Design review of the part built by this model. Coordinates are the model's own, in mm. A direction names the side the tool comes from. Coordinates: 2 decimals unless noted, no trailing zeros. Order: outer loops, then holes, each group sorted by start corner. A loop starts at its lowest first (then second) coordinate and runs counter-clockwise, first axis right, second up. Notation, with made-up numbers: (86, 62.25) -> (104, 62.25) arc R23 ccw to (104, 96.25) -> close; hole circle Ø7 at (6.25, -15). An arc over 180 degrees is marked (long way). Use a Markdown table: item, result. Add a question column.
Q1. Machinability: for faces 4 (the face through (-98.827, 0, 8)), 5 (the face through (-91.827, 0, 12)), which of the approach directions +Z, -Z, +X, -X, +Y, -Y give a long, thin tool a straight path to every point of the face, cutting with its end or side? Answer none if there is none.
Q2. Add section C-C (x = -59.5). State the section outline as (y, z) points, then the cut area to 4 significant figures.
Q3. Add section A-A (z = 12.25). State the section outline as (x, y) points, then the cut area to 4 significant figures.
Q4. Wall thickness on probe 1 along X at (y, z) = (1.5, 8); probe 2 along Z at (x, y) = (-71.5, -0.25): over which ranges is each line inside the solid? List them lowest first.
Q5. Insertion check: pin 1 (8 mm diameter, centred on x = -42.5, y = -0.5, fed in from +Z). The pin has a flat end and moves straight along its axis. Give the tip position at first contact, or say it passes through.
Q6. The part is to be moulded in two halves that separate along X. For faces 1 (the face through (-22.827, 0, 8)), 2 (the face through (-61, 0, 0)), 3 (the face through (-72.487, 0, 12)), say which applies: pulls with the +X half, pulls with the -X half, needs draft (parallel to the pull), parting line crosses it, or undercut.
Q7. Add section B-B (y = 6.5). State the section outline as (x, z) points.
from build123d import *

# Parameters (mm, degrees)
F0_W     = 7
F0_H     = 15.5
F0_W_2   = 12.34
F0_W_3   = 44.66
F0_W_4   = 5
F1_DEPTH = 7
F2_DEPTH = 17


with BuildPart() as f1:
    # F0 (on Top) → F1 (new body)
    with BuildSketch(Plane.XY):
        with Locations((-95.327207, 0)):
            Rectangle(F0_W, F0_H)
        with Locations((-85.657207, 0)):
            Rectangle(F0_W_2, F0_H)
        with Locations((-75.987207, 0)):
            Rectangle(F0_W, F0_H)
        with Locations((-50.157207, 0)):
            Rectangle(F0_W_3, F0_H)
        with Locations((-25.327207, 0)):
            Rectangle(F0_W_4, F0_H)
    extrude(amount=F1_DEPTH)

    # F0 (on Top) → F2 (join)
    with BuildSketch(Plane.XY):
        with Locations((-95.327207, 0)):
            Rectangle(F0_W, F0_H)
        with Locations((-75.987207, 0)):
            Rectangle(F0_W, F0_H)
        with Locations((-25.327207, 0)):
            Rectangle(F0_W_4, F0_H)
    extrude(amount=F2_DEPTH)


solid = f1.part
Established:
| question | item | result |
|---|---|---|
| 1 | face 4 | +Z, -Z, -X, +Y, -Y |
| 1 | face 5 | +Z, +Y, -Y |
| 2 | outline | (-7.75, 0) -> (7.75, 0) -> (7.75, 7) -> (-7.75, 7) -> close |
| 2 | area | 108.5 mm^2 |
| 3 | outline | (-98.83, -7.75) -> (-91.83, -7.75) -> (-91.83, 7.75) -> (-98.83, 7.75) -> close; (-79.49, -7.75) -> (-72.49, -7.75) -> (-72.49, 7.75) -> (-79.49, 7.75) -> close; (-27.83, -7.75) -> (-22.83, -7.75) -> (-22.83, 7.75) -> (-27.83, 7.75) -> close |
| 3 | area | 294.5 mm^2 |
| 4 | probe 1 | -98.83 to -91.83, -79.49 to -72.49, -27.83 to -22.83 |
| 4 | probe 2 | 0 to 7 |
| 5 | pin 1 | z = 7 |
| 6 | face 1 | pulls with the +X half |
| 6 | face 2 | needs draft |
| 6 | face 3 | undercut |
| 7 | outline | (-98.83, 0) -> (-22.83, 0) -> (-22.83, 17) -> (-27.83, 17) -> (-27.83, 7) -> (-72.49, 7) -> (-72.49, 17) -> (-79.49, 17) -> (-79.49, 7) -> (-91.83, 7) -> (-91.83, 17) -> (-98.83, 17) -> close |
